```python
from build123d import *

# Parameters (mm, degrees)
SKETCH1_R           = 3.5
BOSS_EXTRUDE1_DEPTH = 200
SKETCH2_R           = 2
CUT_EXTRUDE1_DEPTH  = 15
CUT_EXTRUDE2_START  = -5
SKETCH3_R           = 3.5
SKETCH3_R_2         = 2.5
CUT_EXTRUDE2_DEPTH  = 5
SKETCH4_R           = 1.5
CUT_EXTRUDE3_DEPTH  = 20


with BuildPart() as part:
    # Sketch1 → Boss-Extrude1 (new body)
    with BuildSketch(Plane.XY):
        Circle(SKETCH1_R)
    extrude(amount=BOSS_EXTRUDE1_DEPTH)

    # Sketch2 → Cut-Extrude1 (cut)
    with BuildSketch(Plane(origin=(0, 0, 0), x_dir=(-1, 0, 0), z_dir=(0, 0, -1))):
        Circle(SKETCH2_R)
    extrude(amount=-CUT_EXTRUDE1_DEPTH, mode=Mode.SUBTRACT)

    # Sketch3 → Cut-Extrude2 (cut)
    with BuildSketch(Plane.XY.offset(200).offset(CUT_EXTRUDE2_START)):
        Circle(SKETCH3_R)
        Circle(SKETCH3_R_2, mode=Mode.SUBTRACT)
    extrude(amount=CUT_EXTRUDE2_DEPTH, mode=Mode.SUBTRACT)

    # Sketch4 → Cut-Extrude3 (cut)
    with BuildSketch(Plane.XY.offset(200)):
        Circle(SKETCH4_R)
    extrude(amount=-CUT_EXTRUDE3_DEPTH, mode=Mode.SUBTRACT)


solid = part.part
```
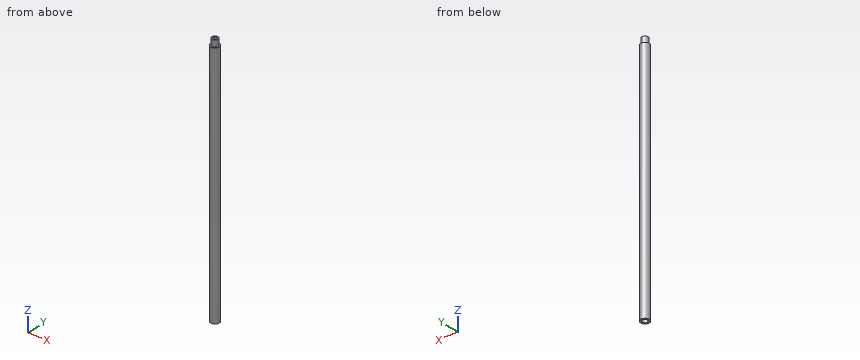
Verification items for the finished model (mm, model axes). Give positions to 0.01 mm unless a question says otherwise; leave off trailing zeros. Order: outer loops, then holes, each group sorted by start corner. A loop starts at its lowest first (then second) coordinate and runs counter-clockwise, first axis right, second up. Notation, with made-up numbers: M 49,17 L 99,17 A19 ccw 99,40 Z; hole C -1,83.25 d10. An arc over 180 degrees is marked long. Answer in a Markdown table with one row per item. Add a question column.
Item 1: Section check C-C, the plane z = 61.5. Enter the section's corners in (x, y).
Item 2: Gauge pin test, flat ends, axial feed: pin 1 (1.5 mm diameter, centred on x = -1, z = 128, fed in from -Y); pin 2 (3 mm diameter, centred on x = -0.5, z = 118.5, fed in from +Y); pin 3 (1.8 mm diameter, centred on x = 0, y = 0, fed in from -Z); pin 4 (1.5 mm diameter, centred on x = -0.5, y = 0.5, fed in from +Z). Record the tip position at first contact, or that the pin passes through.
Item 3: Section check A-A, the plane y = 0. Enter the section's corners in (x, z), and give its area (3 significant figures).
Item 4: Scan lines: probe 1 along Y at (x, z) = (0, 190.25); probe 2 along Z at (x, y) = (1.5, -3); probe 3 along Y at (x, z) = (0, 8.5). Record each from-to range of solid material in increasing order. Write a range as from..to.
Filled sheet:
| question | item | result |
|---|---|---|
| 1 | outline | C 0,0 d7 |
| 2 | pin 1 | stops at y = -3.49 |
| 2 | pin 2 | stops at y = 3.5 |
| 2 | pin 3 | stops at z = 15 |
| 2 | pin 4 | stops at z = 180 |
| 3 | outline | M -3.5,0 L -2,0 L -2,15 L 2,15 L 2,0 L 3.5,0 L 3.5,195 L 2.5,195 L 2.5,200 L 1.5,200 L 1.5,180 L -1.5,180 L -1.5,200 L -2.5,200 L -2.5,195 L -3.5,195 Z |
| 3 | area | 1,270 mm^2 |
| 4 | probe 1 | y = -3.5..-1.5, 1.5..3.5 |
| 4 | probe 2 | z = 0..195 |
| 4 | probe 3 | y = -3.5..-2, 2..3.5 |
